Part model, mm, in its own coordinate system. A direction names the side the tool comes from. Give positions to 0.01 mm unless a question says otherwise; leave off trailing zeros. Order: outer loops, then holes, each group sorted by start corner. A loop starts at its lowest first (then second) coordinate and runs counter-clockwise, first axis right, second up. Notation, with made-up numbers: M 25,31.5 L 52,31.5 A24 cw 52,42.5 Z; hole C 17.25,-31 d10. An arc over 180 degrees is marked long. Answer as a JSON object with one key per item and string values.
from build123d import *

# Parameters (mm, degrees)
RESSALTO_EXTRUS_O1_DEPTH = 4
ESBO_O2_W                = 4
ESBO_O2_H                = 20
CORTE_EXTRUS_O1_DEPTH    = 116.464280191
ESBO_O3_W                = 4
ESBO_O3_H                = 20
CORTE_EXTRUS_O2_DEPTH    = 116.464280191


with BuildPart() as part:
    # Esboço1 → Ressalto-extrusão1 (new body)
    with BuildSketch(Plane.XY):
        Polygon((-50, -100), (-37, -100), (-37, -104), (-13, -104), (-13, -100), (13, -100), (13, -104), (37, -104), (37, -100), (50, -100), (50, 100), (-50, 100), align=None)
    extrude(amount=RESSALTO_EXTRUS_O1_DEPTH)

    # Esboço2 → Corte-extrusão1 (cut, through all)
    with BuildSketch(Plane.XY.offset(4)):
        Polygon((-50, 0), (0, 0), (0, 20), (0, 40), (0, 60), (0, 80), (0, 100), (-50, 100), align=None)
        Polygon((-13, -100), (0, -100), (0, -80), (0, -60), (0, -40), (0, -20), (0, 0), (-50, 0), (-50, -100), (-37, -100), (-37, -104), (-13, -104), align=None)
        with Locations((2, 70)):
            Rectangle(ESBO_O2_W, ESBO_O2_H)
        with Locations((2, -30)):
            Rectangle(ESBO_O2_W, ESBO_O2_H)
        with Locations((2, -70)):
            Rectangle(ESBO_O2_W, ESBO_O2_H)
        with Locations((2, 30)):
            Rectangle(ESBO_O2_W, ESBO_O2_H)
    extrude(amount=-CORTE_EXTRUS_O1_DEPTH, mode=Mode.SUBTRACT)

    # Esboço3 → Corte-extrusão2 (cut, through all)
    with BuildSketch(Plane.XY.offset(4)):
        with Locations((48, 70)):
            Rectangle(ESBO_O3_W, ESBO_O3_H)
        with Locations((48, 30)):
            Rectangle(ESBO_O3_W, ESBO_O3_H)
        with Locations((48, -70)):
            Rectangle(ESBO_O3_W, ESBO_O3_H)
        with Locations((48, -30)):
            Rectangle(ESBO_O3_W, ESBO_O3_H)
    extrude(amount=-CORTE_EXTRUS_O2_DEPTH, mode=Mode.SUBTRACT)


solid = part.part
1. Two-plate mould, pull along Y, no slides. Class faces 4 (the flat face through (2, -80, 2)), 5 (the flat face through (0, 50, 2)): +Y half, -Y half, draft (parallel to the pull), parting line (faces both ways), or undercut.
Worked answers:
{"face 4": "undercut", "face 5": "draft"}
2. Cut at B-B on x = 8. Give the cut face in (y, z).
Worked answers:
{"outline": "M -100,0 L 100,0 L 100,4 L -100,4 Z"}
3. Pin check, flat tips, straight feed: P1, Ø1.2, axis at x = 48, z = 2.5, coming from the -Y side; P2, Ø2, axis at x = 37, y = -56.5, coming from the -Z side; P3, Ø2, axis at y = -102.5, z = 3, coming from the +X side. Stop position of each tip, or through.
Worked answers:
{"P1": "stops at y = -100", "P2": "stops at z = 0", "P3": "stops at x = 37"}
4. Probe line 1 along Y through (x, z) = (48, 1.75); line 2 along Y through (x, z) = (8, 1.6); line 3 along X through (y, z) = (-32.5, 0.25). List the from-to ranges inside material, lowest first.
Worked answers:
{"line 1": "y = -100 to -80, -60 to -40, -20 to 20, 40 to 60, 80 to 100", "line 2": "y = -100 to 100", "line 3": "x = 4 to 46"}
5. Which spindle directions (+Z, -Z, +X, -X, +Y, -Y) get a long thin tool onto all of the face, cutting with end or side? Do faces 1 (the flat face through (2, 40, 2)), 2 (the flat face through (37, -102, 2)), 3 (the flat face through (46, 30, 2)). Say none if no direction does.
Worked answers:
{"face 1": "+Z, -Z, -X", "face 2": "+Z, -Z, +X, -Y", "face 3": "+Z, -Z, +X"}
6. Cut at A-A on y = 34. Give the cut face in (x, z), plus the area to 3 significant figures.
Worked answers:
{"outline": "M 4,0 L 46,0 L 46,4 L 4,4 Z", "area": "168 mm^2"}
